Read the model definition and answer for the solid it produces. Units are mm, in the model's axes. A direction names the side the tool comes from. Round coordinates to 2 decimals unless told otherwise and drop trailing zeros. Write each loop counter-clockwise with the first axis right and the second up, starting at its lowest first coordinate (ties: lowest second). Pieces come first, ordered by that corner, then holes. Notation, with made-up numbers: (34, -18) - (91, -18) arc R15 ccw to (91, 6) - close; hole circle Ø9 at (-34.5, 72.25). An arc over 180 degrees is marked (long way). Answer as CSV lines item,"result". Start each with the question number.
1) Each of these flat-tipped pins is pushed along its axis until it touches: pin 1 (3 mm diameter, centred on y = 4, z = 6.5, fed in from +X); pin 2 (5 mm diameter, centred on x = 8.5, z = 5.5, fed in from -Y); pin 3 (5 mm diameter, centred on x = 8.5, y = 3, fed in from +Z); pin 4 (1.8 mm diameter, centred on x = 12.98, z = 3.3, fed in from -Y). Where does it stop, or does it pass through?
2) Which of the six approach directions +Z, -Z, +X, -X, +Y, -Y give full straight-line access (tool end or side, diameter ignored) to faces 1 (the flat face through (-4, 0.83, 3)), 2 (the flat face through (18.326, -7, 3)), 3 (the flat face through (1.846, 5, 3)), 4 (the flat face through (23.798, -7, 3)), 5 (the cylindrical face through (14.4, -1.49, 3.88))?
3) Consider line 1 along X through (y, z) = (-4, 0.5); line 2 along X through (y, z) = (2, 3); line 3 along Y through (x, z) = (0, -0.5). Determine where each line is inside the solid, lowest interval first.
4) Find section C-C on z = 4. State how many separate pieces and enclosed holes the cut face has, then the cut area to 3 significant figures.
5) Find section D-D on x = 3.5. Determine the outline of the cut face in (y, z) (3 decimals), then the cut area to 3 significant figures.
6) Find section A-A on y = 1.75. Determine the outline of the cut face in (x, z), then the cut area to 3 significant figures.
7) For a pull along Z with two mould halves and no side action, classify faces 6 (the flat face through (14.7, -3.7, -1.785)), 7 (the flat face through (9.196, 4, 3)), 8 (the flat face through (21, -3.72, 3)) as +Z half, -Z half, draft (parallel to the pull), parting line (faces both ways), or undercut.
8) Find section B-B on y = -9.75. Determine the outline of the cut face in (x, z) (3 decimals).
Autodesk Inventor part; units mm, degrees
ref_plane "YZ Plane" through (0, 0, 0) normal (1, 0, 0) x (0, 1, 0)
ref_plane "XZ Plane" through (0, 0, 0) normal (0, 1, 0) x (-1, 0, 0)
ref_plane "XY Plane" through (0, 0, 0) normal (0, 0, 1) x (1, 0, 0)
sketch "Sketch1" plane through (0, 0, 0) normal (0, 0, 1) x (1, 0, 0)
  line L0 (-8.7842, -2.2796) -> (15.8158, -2.2796)
  line L1 (15.8158, -2.2796) -> (15.8158, 0.8304)
  line L2 (15.8158, 0.8304) -> (9.1958, 0.8304)
  line L3 (9.1958, 0.8304) -> (9.1958, 7.7401)
  line L4 (9.1958, 7.7401) -> (8.2439, 8.6704)
  line L5 (8.2439, 8.6704) -> (4.8058, 8.6704)
  line L6 (4.8058, 8.6704) -> (4.8058, 0.8304)
  line L7 (4.8058, 0.8304) -> (1.8458, 0.8304)
  line L8 (1.8458, 0.8304) -> (1.8458, 8.6704)
  line L9 (1.8458, 8.6704) -> (-2.6742, 8.6704)
  line L10 (-2.6742, 8.6704) -> (-2.6742, 0.8304)
  line L11 (-2.6742, 0.8304) -> (-8.7842, 0.8304)
  line L12 (-8.7842, 0.8304) -> (-8.7842, -2.2796)
  point P0 (0, 0)
  dimension "d0" = 24.6
  dimension "d1" = 3.11
  dimension "d2" = 4.39
  dimension "d3" = 2.96
  dimension "d4" = 4.52
  dimension "d5" = 6.62
  dimension "d6" = 7.84
extrude "Extrusion1" add sketch "Sketch1" along normal blind 6.43
sketch "Sketch2" plane through (9.1958, 0.8304, 0) normal (0, 1, 0) x (1, 0, 0)
  line L0 (6.62, 0) -> (0, 0)
  line L1 (6.62, -6.43) -> (0, -6.43)
  line L2 (6.62, 0) -> (6.62, -6.43) construction
  line L3 (6.62, -4.83) -> (-18.0124, -4.83) construction
  line L4 (-18.0124, -1.76) -> (6.62, -1.76) construction
  line L5 (-17.98, 0) -> (-17.98, -6.43) construction
  line L6 (-11.87, 0) -> (-17.98, 0) construction
  line L7 (-11.87, -6.43) -> (-17.98, -6.43) construction
  line L8 (-16.68, -6.43) -> (-16.68, 0) construction
  circle A0 centre (-15.145, -3.295) radius 1.535
  line L9 (5.32, 0) -> (5.32, -6.43) construction
  circle A1 centre (3.785, -3.295) radius 1.535
  point P0 (-9.1958, 0)
  dimension "d9" = 1.76
  dimension "d10" = 1.6
  dimension "d11" = 1.3
  dimension "d12" = 1.3
extrude "Extrusion2" cut sketch "Sketch2" along normal up to surface (3.11 mm away) from surface at -3.11
sketch "Sketch3" plane through (-8.7842, -2.2796, 0) normal (0, -1, 0) x (1, 0, 0)
  circle A0 centre (2.835, 3.295) radius 1.535
  circle A1 centre (21.765, 3.295) radius 1.535
  line L0 (0, 0) -> (0, 6.43)
  line L1 (0, -1.785) -> (32.89, -1.785)
  line L2 (32.89, -1.785) -> (32.89, 8.215)
  line L3 (32.89, 8.215) -> (0, 8.215)
  line L4 (0, 8.215) -> (0, -1.785)
  line L5 (0, 3.215) -> (32.89, 3.215) construction
  point P0 (8.7842, 0)
  dimension "d15" = 32.89
  dimension "d16" = 10
extrude "Extrusion3" add sketch "Sketch3" along normal blind 1.6
sketch "Sketch4" plane through (-8.7842, -3.8796, 0) normal (0, -1, 0) x (1, 0, 0)
  line L0 (0, -1.785) -> (32.89, -1.785)
  line L1 (32.89, 8.215) -> (27.11, 8.215)
  line L2 (27.11, 8.215) -> (27.11, -1.785)
  line L3 (27.11, -1.785) -> (32.89, -1.785)
  line L4 (32.89, -1.785) -> (32.89, 8.215)
  point P0 (8.7842, 0)
  dimension "d19" = 5.78
extrude "Extrusion4" add sketch "Sketch4" along normal blind 7.17
sketch "Sketch5" plane through (-8.7842, -11.0496, 0) normal (0, -1, 0) x (1, 0, 0)
  line L0 (27.5471, -1.3186) -> (32.5822, -1.3186)
  line L1 (32.5822, -1.3186) -> (32.5822, 7.8489)
  line L2 (32.5822, 7.8489) -> (27.5471, 7.8489)
  line L3 (27.5471, 7.8489) -> (27.5471, -1.3186)
  point P0 (8.7842, 0)
extrude "Extrusion5" cut sketch "Sketch5" against normal blind 7.33
properties part number "optical stop"
Check values:
1,pin 1,"stops at x = 9.2"
1,pin 2,"stops at y = -3.88"
1,pin 3,"stops at z = 6.43"
1,pin 4,"passes through"
2,face 1,"+Z, -Z, -X, +Y"
2,face 2,"+Z, -Z, -X, -Y"
2,face 3,"+Z, -Z, +Y"
2,face 4,"-Y"
2,face 5,"+Y, -Y"
3,line 1,"x = 18.33 to 18.76, 23.8 to 24.11"
3,line 2,"x = -2.67 to 1.85, 4.81 to 9.2"
3,line 3,"y = -3.88 to -2.28"
4,separate pieces,"3"
4,enclosed holes,"0"
4,area,"177 mm^2"
5,outline,"(-3.88, -1.785) - (-2.28, -1.785) - (-2.28, 0) - (0.83, 0) - (0.83, 6.43) - (-2.28, 6.43) - (-2.28, 8.215) - (-3.88, 8.215) - close"
5,area,"36.0 mm^2"
6,outline,"(-2.67, 0) - (1.85, 0) - (1.85, 6.43) - (-2.67, 6.43) - close; (4.81, 0) - (9.2, 0) - (9.2, 6.43) - (4.81, 6.43) - close"
6,area,"57.3 mm^2"
7,face 6,"-Z half"
7,face 7,"draft"
7,face 8,"undercut"
8,outline,"(18.326, -1.785) - (24.106, -1.785) - (24.106, 8.215) - (18.326, 8.215) - close; hole (18.763, -1.319) - (23.798, -1.319) - (23.798, 7.849) - (18.763, 7.849) - close"
